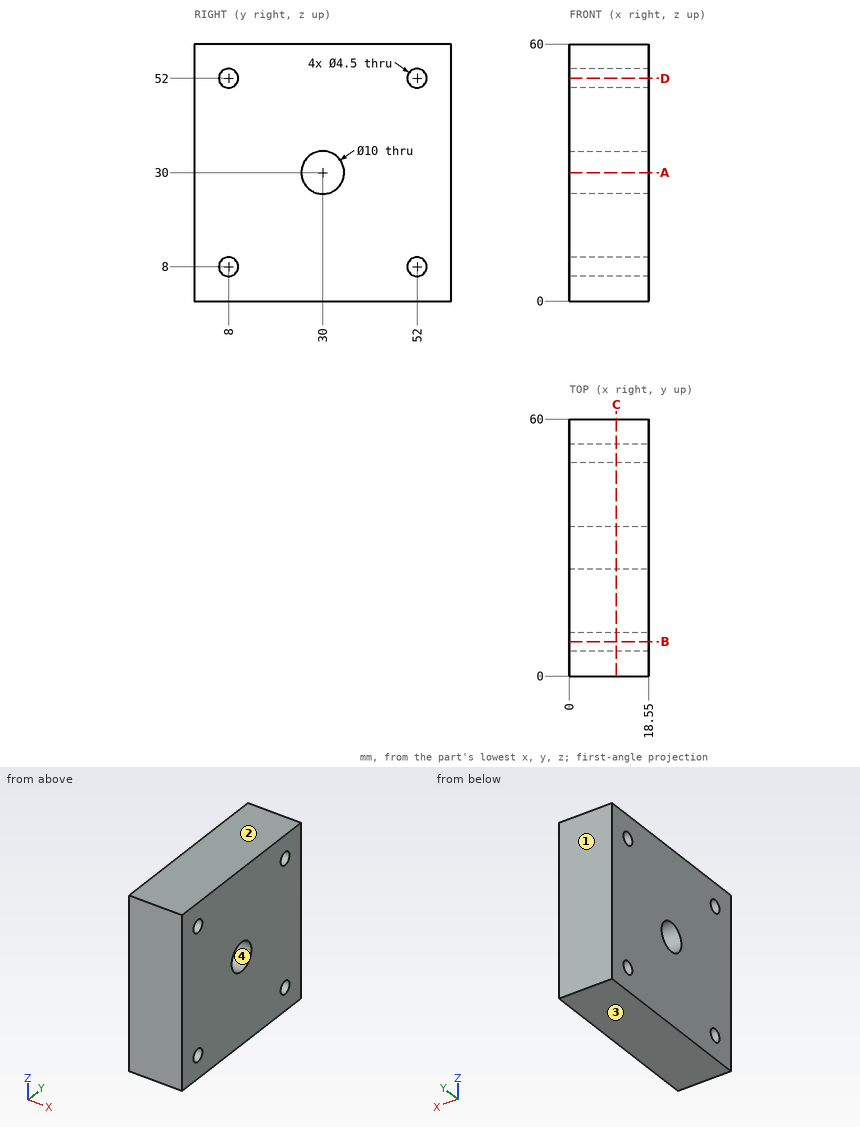
Part print with two shaded views. Sizes in mm from the minimum x, y, z corner. Round coordinates to 2 decimals unless told otherwise and drop trailing zeros. Loops run counter-clockwise (first coordinate to the right, second up) from the corner with the lowest first, then second, coordinate; pieces in that order, holes last.
Item 1: Drill centre lines: line 1 along Z through (x, y) = (13.75, 52); line 2 along Z through (x, y) = (5.25, 34.5); line 3 along Y through (x, z) = (14.75, 27.5). Where is each one in solid material? Low to high.
Item 2: Saw through at C-C (x = 11). List the corners of the cut face in (y, z).
Item 3: Saw through at A-A (z = 30). List the corners of the cut face in (x, y).
Item 4: Pin check, flat tip, straight feed: P1, Ø7, axis at y = 52, z = 52, coming from the +X side. Stop position of the tip, or through.
Item 5: Saw through at B-B (y = 8). List the corners of the cut face in (x, z), then the cut area to 3 significant figures.
Item 6: Two-plate mould, pull along Z, no slides. Class the marked faces 1, 2, 3 and 4: released by +Z, released by -Z, zero draft, split by the parting line, or undercut.
Worked answers:
1. line 1: z = 0 to 5.75, 10.25 to 49.75, 54.25 to 60
1. line 2: z = 0 to 27.82, 32.18 to 60
1. line 3: y = 0 to 25.67, 34.33 to 60
2. outline: (0, 0) - (60, 0) - (60, 60) - (0, 60) - close; hole circle Ø4.5 at (8, 8); hole circle Ø4.5 at (8, 52); hole circle Ø10 at (30, 30); hole circle Ø4.5 at (52, 8); hole circle Ø4.5 at (52, 52)
3. outline: (0, 0) - (18.55, 0) - (18.55, 25) - (0, 25) - close; (0, 35) - (18.55, 35) - (18.55, 60) - (0, 60) - close
4. P1: stops at x = 18.55
5. outline: (0, 0) - (18.55, 0) - (18.55, 5.75) - (0, 5.75) - close; (0, 10.25) - (18.55, 10.25) - (18.55, 49.75) - (0, 49.75) - close; (0, 54.25) - (18.55, 54.25) - (18.55, 60) - (0, 60) - close
5. area: 946 mm2
6. face 1: zero draft
6. face 2: released by +Z
6. face 3: released by -Z
6. face 4: undercut
